Autodesk Inventor part; units mm, degrees
ref_plane "YZ Plane" through (0, 0, 0) normal (1, 0, 0) x (0, 1, 0)
ref_plane "XZ Plane" through (0, 0, 0) normal (0, 1, 0) x (-1, 0, 0)
ref_plane "XY Plane" through (0, 0, 0) normal (0, 0, 1) x (1, 0, 0)
sketch "Эскиз1" plane through (0, 0, 0) normal (0, 0, 1) x (1, 0, 0)
  circle A0 centre (0, 98.9661) radius 2
  circle A1 centre (0, -0.7112) radius 2
  line L0 (-22, 101.1274) -> (22, 101.1274)
  line L1 (22, 101.1274) -> (22, -2.8726)
  line L2 (22, -2.8726) -> (-22, -2.8726)
  line L3 (-22, -2.8726) -> (-22, 101.1274)
  line L4 (21.7, 100.8274) -> (-21.7, 100.8274)
  line L5 (-21.7, 100.8274) -> (-21.7, -2.5726)
  line L6 (-21.7, -2.5726) -> (21.7, -2.5726)
  line L7 (21.7, -2.5726) -> (21.7, 100.8274)
  point P0 (0, 0)
  point P1 (-0.7318, -2.5726)
  point P2 (0.7318, -2.5726)
  point P3 (0.7318, 100.8274)
  point P4 (-0.7318, 100.8274)
  dimension "d0" = 0.3
  dimension "d1" = 0.3
  dimension "d2" = 0.3
  dimension "d3" = 0.3
extrude "Выдавливание1" add sketch "Эскиз1" along normal blind 3.5 contours A0 L4 L7 L6 A1 L5
sketch "Эскиз2" plane through (0, 0, 3.5) normal (0, 0, 1) x (1, 0, 0)
  line L0 (-21.7, -2.5726) -> (-0.7318, -2.5726)
  arc A0 (0.7318, -2.5726) -> (-0.7318, -2.5726) centre (0, -0.7112) ccw
  line L1 (0.7318, -2.5726) -> (21.7, -2.5726)
  line L2 (21.7, -2.5726) -> (21.7, 100.8274)
  line L3 (21.7, 100.8274) -> (0.7318, 100.8274)
  arc A1 (-0.7318, 100.8274) -> (0.7318, 100.8274) centre (0, 98.9661) ccw
  line L4 (-0.7318, 100.8274) -> (-21.7, 100.8274)
  line L5 (-21.7, 100.8274) -> (-21.7, -2.5726)
  arc A2 (-0.7318, 100.8274) -> (0.7318, 100.8274) centre (0, 98.9661) ccw
  arc A3 (0.7318, -2.5726) -> (-0.7318, -2.5726) centre (0, -0.7112) ccw
  line L6 (0, 98.9661) -> (0, -0.7112)
  line L7 (4.3137, 74.1274) -> (-5.6863, 74.1274)
  line L8 (-5.6863, 74.1274) -> (-5.6863, 24.1274)
  line L9 (-5.6863, 24.1274) -> (4.3137, 24.1274)
  line L10 (4.3137, 24.1274) -> (4.3137, 74.1274)
  point P0 (0, 0)
  dimension "d6" = 10
  dimension "d7" = 50
  dimension "d8" = 103.4
  dimension "d9" = 26.7
extrude "Выдавливание2" add sketch "Эскиз2" along normal blind 10 contours L9 L8 L7 L6 | L6 L7 L10 L9
sketch "Эскиз3" plane through (-5.6863, 74.1274, 3.5) normal (0, 1, 0) x (1, 0, 0)
  line L0 (0, 0) -> (0, -10)
  line L1 (4.9545, 0) -> (-16.0137, 0)
  arc A0 (0, -10) -> (-0.0123, 0) centre (-9.3916, -5.0116) ccw
  line L2 (10, -10) -> (0, -10)
  line L3 (5, -12.0906) -> (5, 6.7336) construction
  line L4 (7.6863, 0) -> (3.6863, 0)
  line L5 (10, 0) -> (10, -10)
  arc A1 (10.0123, 0) -> (10, -10) centre (19.3916, -5.0116) ccw
  point P0 (5.6863, 3.5)
  point P1 (6.418, 0)
  point P2 (0, -0.0232)
  point P3 (10, -0.0232)
extrude "Выдавливание3" cut sketch "Эскиз3" against normal blind 58.75 contours A1 L5 | A0 L0
fillet "Сопряжение1" radius 2 2 edges at (4.3137, 49.1274, 13.5) (-5.6863, 49.1274, 13.5)
fillet "Сопряжение2" radius 2 10 edges at (-4.5263, 74.1274, 7.1886) (-0.6863, 74.1274, 13.5) (3.0022, 74.1274, 12.7357) (3.1537, 74.1274, 7.1886) (-4.3748, 74.1274, 12.7357) (-0.6863, 24.1274, 13.5) (3.0022, 24.1274, 12.7357) (3.1537, 24.1274, 7.1886) (-4.5263, 24.1274, 7.1886) (-4.3748, 24.1274, 12.7357)
equation "\"d0\" = d1"
equation "\"d2\" = d0"
equation "\"d3\" = d0"
equation "\"d9\" = -0.5 * d7 + 0.5 * d8"
properties part number "battery_case_top"
Input: part model. Units: mm. Frame: model coordinates. A direction names the side the tool comes from. Give positions to 0.01 mm unless a question says otherwise; leave off trailing zeros. Loops run counter-clockwise (first coordinate to the right, second up) from the corner with the lowest first, then second, coordinate; pieces in that order, holes last. Notation, with made-up numbers: (11.5, 28) -> (69.5, 28) arc R30 cw to (69.5, 66) -> close; hole circle Ø7 at (35.5, 68). An arc over 180 degrees is marked (long way). Answer as a JSON object with one key per item and string values. Group by question number.
Item 1: Cut plane C-C, the plane x = 18.5. Return the cut outline in (y, z), and give its area (3 significant figures).
Item 2: Pull-direction query (X, two-part tool) for faces 1 (the flat face through (-1, 49, 13.5)), 2 (the cylindrical face through (0.077, 96.968, 1.726)), 3 (the cylindrical face through (2.986, 49.449, 12.756)); classes: released by +X, released by -X, zero draft, split by the parting line, or undercut.
Item 3: Cut plane B-B, the plane z = 12.5. Return the cut outline in (x, y), and give its area (3 significant figures).
Item 4: Reachability of faces 4 (the flat face through (0, 50, 0)), 5 (the flat face through (-1, 74.127, 7)), 6 (the flat face through (-1, 24.127, 7)) from +Z, -Z, +X, -X, +Y, -Y: full face, straight path, thin tool, end or side. Return the list, or none.
Item 5: Pin query (flat end, axial travel): P1, Ø3, axis at x = 15.5, y = 87, coming from the +Z side; P2, Ø3, axis at x = 0, y = 98.97, coming from the +Z side; P3, Ø1.7, axis at x = 0.5, z = 6.5, coming from the -Y side; P4, Ø13, axis at x = 9.5, y = 56, coming from the +Z side. Return the tip coordinate at first contact, or that it passes through.
Item 6: Line query: probe 1 along Z at (x, y) = (12.5, 83); probe 2 along Y at (x, z) = (0, 1.8); probe 3 along X at (y, z) = (27, 12.25). Output: solid intervals per line, ascending.
Item 7: Cut plane D-D, the plane y = 11. Return the cut outline in (x, z).
Checks:
{
 "1": {"outline": "(-2.57, 0) -> (100.83, 0) -> (100.83, 3.5) -> (-2.57, 3.5) -> close", "area": "362 mm²"},
 "2": {"face 1": "zero draft", "face 2": "undercut", "face 3": "released by +X"},
 "3": {"outline": "(-4.53, 26.13) arc R1.73 ccw to (-2.8, 24.4) -> (1.43, 24.4) arc R1.73 ccw to (3.16, 26.13) -> (3.16, 72.13) arc R1.73 ccw to (1.43, 73.86) -> (-2.8, 73.86) arc R1.73 ccw to (-4.53, 72.13) -> close", "area": "378 mm²"},
 "4": {"face 4": "-Z, +X, -X, +Y, -Y", "face 5": "+Z, +X, -X, +Y", "face 6": "+Z, +X, -X, -Y"},
 "5": {"P1": "stops at z = 3.5", "P2": "passes through", "P3": "stops at y = 24.13", "P4": "stops at z = 12.74"},
 "6": {"probe 1": "z = 0 to 3.5", "probe 2": "y = 1.29 to 96.97", "probe 3": "x = -4.66 to 3.28"},
 "7": {"outline": "(-21.7, 0) -> (21.7, 0) -> (21.7, 3.5) -> (-21.7, 3.5) -> close"}
}
